Design review of the part shown in the three views and the two pictorial views. Dimensions are in mm from the part's minimum x, y and z. A direction names the side the tool comes from. Coordinates: 2 decimals unless noted, no trailing zeros. Order: outer loops, then holes, each group sorted by start corner. A loop starts at its lowest first (then second) coordinate and runs counter-clockwise, first axis right, second up. Notation, with made-up numbers: (52, 86) -> (62, 86) arc R27 cw to (62, 104) -> close; hole circle Ø8 at (-24.75, 18.25). An arc over 180 degrees is marked (long way). Answer as CSV lines item,"result". Start each with the question number.
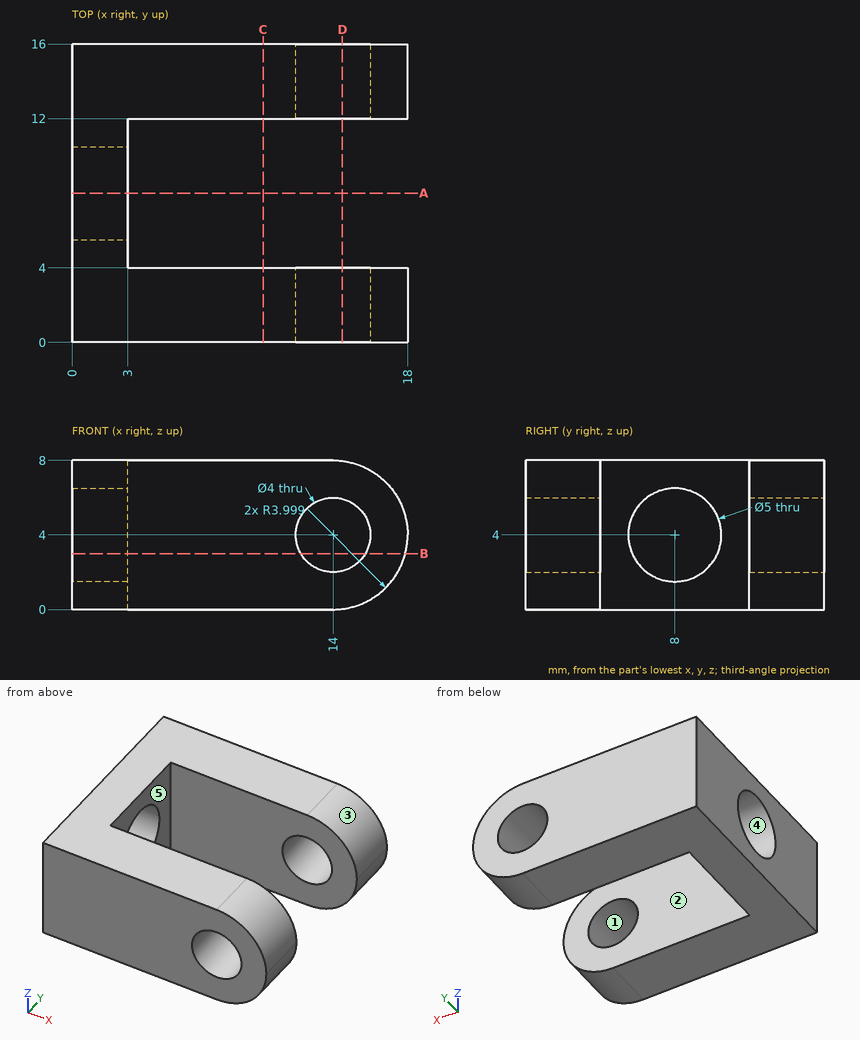
1) Mouldability with a two-part tool opening along Z and no side actions: class the marked faces 1, 2 and 3 as released by +Z, released by -Z, zero draft, split by the parting line, or undercut.
2) Tool access review of the marked faces 4 and 5: name each direction out of +Z, -Z, +X, -X, +Y, -Y from which nothing blocks a thin tool from reaching the whole face with its end or side.
3) Insertion check: pin 1 Ø4 at (y, z) = (7, 2.5) entering from +X. The pin has a flat end and moves straight along its axis. Give the tip position at first contact, or say it passes through.
4) Consider section A-A (y = 8). Give the boundary of the cut face in (x, z).
5) Consider section D-D (x = 14.5). Give the boundary of the cut face in (y, z).
6) Consider section B-B (z = 3). Give the boundary of the cut face in (x, y).
7) Wall thickness on L1, parallel to Z at x = 14, y = 13.05; L2, parallel to X at y = 2.95, z = 4; L3, parallel to Y at x = 9.75, z = 3.5: over which ranges is each line inside the solid? List them lowest first. Write a range as [from, to].
8) Consider section C-C (x = 10.25). Give the boundary of the cut face in (y, z).
Result:
1,face 1,"undercut"
1,face 2,"zero draft"
1,face 3,"released by +Z"
2,face 4,"+X, -X"
2,face 5,"+Z, -Z, +X"
3,pin 1,"x = 3"
4,outline,"(0, 0) -> (3, 0) -> (3, 1.5) -> (0, 1.5) -> close; (0, 6.5) -> (3, 6.5) -> (3, 8) -> (0, 8) -> close"
5,outline,"(0, 0.03) -> (4, 0.03) -> (4, 2.06) -> (0, 2.06) -> close; (0, 5.94) -> (4, 5.94) -> (4, 7.97) -> (0, 7.97) -> close; (12, 0.03) -> (16, 0.03) -> (16, 2.06) -> (12, 2.06) -> close; (12, 5.94) -> (16, 5.94) -> (16, 7.97) -> (12, 7.97) -> close"
6,outline,"(0, 0) -> (12.27, 0) -> (12.27, 4) -> (3, 4) -> (3, 5.71) -> (0, 5.71) -> close; (0, 10.29) -> (3, 10.29) -> (3, 12) -> (12.27, 12) -> (12.27, 16) -> (0, 16) -> close; (15.73, 0) -> (17.87, 0) -> (17.87, 4) -> (15.73, 4) -> close; (15.73, 12) -> (17.87, 12) -> (17.87, 16) -> (15.73, 16) -> close"
7,L1,"[0, 2], [6, 8]"
7,L2,"[0, 12], [16, 18]"
7,L3,"[0, 4], [12, 16]"
8,outline,"(0, 0) -> (4, 0) -> (4, 8) -> (0, 8) -> close; (12, 0) -> (16, 0) -> (16, 8) -> (12, 8) -> close"
